Geometry check sheet. Reference: the model listing, model coordinates, mm. Face numbers are marked on the shaded views. A direction names the side the tool comes from. Give positions to 0.01 mm unless a question says otherwise; leave off trailing zeros. Loops run counter-clockwise (first coordinate to the right, second up) from the corner with the lowest first, then second, coordinate; pieces in that order, holes last. Notation, with made-up numbers: (-4.75, -9.5) - (43.25, -9.5) arc R29 ccw to (43.25, 17.5) - close; hole circle Ø11 at (-15.75, -19). An arc over 180 degrees is marked (long way). Write item = value, one per line. Start each with the question number.
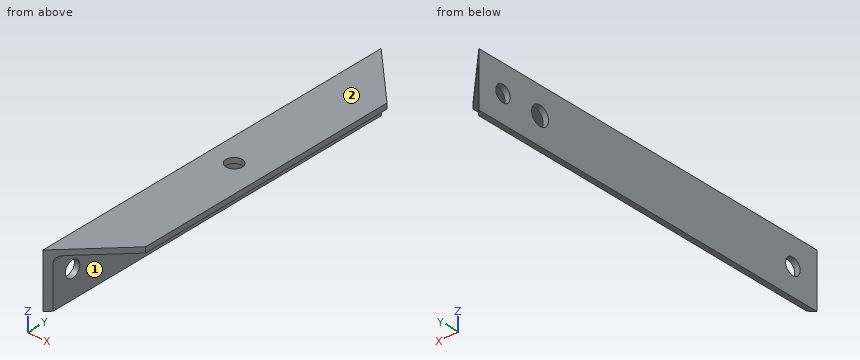
from build123d import *

# Parameters (mm, degrees)
F1_DEPTH = 210
F3_D     = 9
F3_DEPTH = 12
F3_TIP   = 2.7038727856
F5_D     = 10.5
F5_DEPTH = 12
F5_TIP   = 3.1545182499
F7_D     = 9
F7_DEPTH = 12
F7_TIP   = 2.7038727856
F9_DEPTH = 94


with BuildPart() as f1:
    # F0 (on Front) → F1 (new body)
    with BuildSketch(Plane.XZ):
        with BuildLine():
            Line((0, 30), (0, 0))
            Line((0, 0), (3, 0))
            Line((3, 0), (3, 24))
            ThreePointArc((3, 24), (3.8786796564, 26.1213203436), (6, 27))
            Line((6, 27), (30, 27))
            Line((30, 27), (30, 30))
            Line((30, 30), (0, 30))
        make_face()
    extrude(amount=F1_DEPTH)

    # F3
    with Locations(Plane.YZ.offset(3)):
        with Locations((-195, 15), (-15, 15)):
            Hole(F3_D / 2, depth=F3_DEPTH)
            with Locations((0, 0, -(F3_DEPTH + F3_TIP / 2))):  # 118° drill point
                Cone(0, F3_D / 2, F3_TIP, mode=Mode.SUBTRACT)

    # F5
    with Locations(Plane.YZ.offset(3)):
        with Locations((-38, 15)):
            Hole(F5_D / 2, depth=F5_DEPTH)
            with Locations((0, 0, -(F5_DEPTH + F5_TIP / 2))):  # 118° drill point
                Cone(0, F5_D / 2, F5_TIP, mode=Mode.SUBTRACT)

    # F7
    with Locations(Plane(origin=(0, 0, 27), x_dir=(1, 0, 0), z_dir=(0, 0, -1))):
        with Locations((14, 107)):
            Hole(F7_D / 2, depth=F7_DEPTH)
            with Locations((0, 0, -(F7_DEPTH + F7_TIP / 2))):  # 118° drill point
                Cone(0, F7_D / 2, F7_TIP, mode=Mode.SUBTRACT)

    # F8 (on face) → F9 (cut)
    with BuildSketch(Plane(origin=(0, 0, 0), x_dir=(1, 0, 0), z_dir=(0, 0, -1))):
        Polygon((30, 30), (3, 3), (3, 0), (30, 0), align=None)
        Polygon((3, 210), (3, 207), (30, 180), (30, 210), align=None)
        Polygon((3, 3), (0, 0), (3, 0), align=None)
        Polygon((3, 210), (0, 210), (3, 207), align=None)
    extrude(amount=-F9_DEPTH, mode=Mode.SUBTRACT)


solid = f1.part
1) Tool access check on the marked faces 1 and 2. Record the directions out of +Z, -Z, +X, -X, +Y, -Y that give a thin tool (end or side, any length) a straight path to the whole face; none if there is none.
2) Cross-section at A-A on y = -38. Enter the section's corners in (x, z).
3) Gauge pin test, flat ends, axial feed: P1, Ø12, axis at x = 12, y = -102, coming from the -Z side; P2, Ø5, axis at x = 5, z = 18, coming from the +Y side; P3, Ø12, axis at y = -84, z = 12, coming from the +X side. Record the tip position at first contact, or that the pin passes through.
4) Cross-section at B-B on x = 14. Enter the section's corners in (y, z), and give its area (3 significant figures).
5) Cross-section at C-C on y = -166. Enter the section's corners in (x, z).
6) Cross-section at D-D on z = 6.5. Enter the section's corners in (x, y), and give its area (3 significant figures).
7) Material ranges on line 1 along Z through (x, y) = (2, -195); line 2 along X through (y, z) = (-107, 28); line 3 along Z through (x, y) = (27, -46), recorded low to high.
Checked values:
q1.face_1 = -Z, +X, +Y, -Y
q1.face_2 = +Z, +X, -X, +Y, -Y
q2.outline = (0, 0) - (3, 0) - (3, 9.75) - (0, 9.75) - close; (0, 20.25) - (3, 20.25) - (3, 24) arc R3 cw to (6, 27) - (30, 27) - (30, 30) - (0, 30) - close
q3.P1 = 27
q3.P2 = -2.5
q3.P3 = 3
q4.outline = (-196, 27) - (-111.5, 27) - (-111.5, 30) - (-196, 30) - close; (-102.5, 27) - (-14, 27) - (-14, 30) - (-102.5, 30) - close
q4.area = 519 mm²
q5.outline = (0, 0) - (3, 0) - (3, 24) arc R3 cw to (6, 27) - (30, 27) - (30, 30) - (0, 30) - close
q6.outline = (0, -210) - (3, -207) - (3, -3) - (0, 0) - close
q6.area = 621 mm²
q7.line_1 = 0 to 10.5, 19.5 to 30
q7.line_2 = 0 to 9.5, 18.5 to 30
q7.line_3 = 27 to 30
